CAD build for the part. Positions are in the model's coordinates, mm. Face numbers are marked on the shaded views. A direction names the side the tool comes from. Give positions to 0.01 mm unless a question says otherwise; leave off trailing zeros. Loops run counter-clockwise (first coordinate to the right, second up) from the corner with the lowest first, then second, coordinate; pieces in that order, holes last. Notation, with made-up numbers: (67, 50.5) -> (72, 50.5) arc R24 cw to (72, 61.5) -> close; hole circle Ø3 at (-4.75, 49.5). An arc over 180 degrees is marked (long way). Use one line per item in the form item = value.
```python
from build123d import *

# Parameters (mm, degrees)
CUT_EXTRUDE1_START         = -1.5875
CUT_EXTRUDE1_OUTLINE_W     = 53.975
CUT_EXTRUDE1_OUTLINE_H     = 19.05
CUT_EXTRUDE1_OUTLINE_W_2   = 50.8
CUT_EXTRUDE1_OUTLINE_H_2   = 15.875
CUT_EXTRUDE1_DEPTH         = 38.1
CUT_EXTRUDE1_START_2       = 30.1625
CUT_EXTRUDE1_2_DEPTH       = 166.6875
CUT_EXTRUDE1_3_DEPTH       = 6.35
CUT_EXTRUDE1_4_OUTLINE_W   = 50.8
CUT_EXTRUDE1_4_OUTLINE_H   = 15.875
CUT_EXTRUDE1_4_OUTLINE_W_2 = 7.9375
CUT_EXTRUDE1_4_OUTLINE_H_2 = 12.7
CUT_EXTRUDE1_4_DEPTH       = 1.5875
CUT_EXTRUDE1_5_DEPTH       = 26.9875
CUT_EXTRUDE1_6_OUTLINE_W   = 28.575
CUT_EXTRUDE1_6_OUTLINE_H   = 19.05
CUT_EXTRUDE1_6_DEPTH       = 7.9375
CUT_EXTRUDE1_START_3       = 2.38125
CUT_EXTRUDE1_7_DEPTH       = 14.2875
CUT_EXTRUDE1_8_DEPTH       = 19.05
SKETCH2_W                  = 8.89
SKETCH2_H                  = 2.5908
CUT_EXTRUDE2_DEPTH         = 203.030816028
SKETCH3_W                  = 1.9812
SKETCH3_H                  = 2.9972
CUT_EXTRUDE3_DEPTH         = 203.030816028
FILLET1_R                  = 1.5875
HOLE1_D                    = 6.35
HOLE1_DEPTH                = 1.5875


with BuildPart() as part:
    # Cut-Extrude1: read off the stored shape, not the designer's step
    # Cut-Extrude1 outline → Cut-Extrude1 (new body)
    with BuildSketch(Plane.XY.offset(-36.5125).offset(CUT_EXTRUDE1_START)):
        with Locations((14.2875, 9.525)):
            Rectangle(CUT_EXTRUDE1_OUTLINE_W, CUT_EXTRUDE1_OUTLINE_H)
        with Locations((14.2875, 9.525)):
            Rectangle(CUT_EXTRUDE1_OUTLINE_W_2, CUT_EXTRUDE1_OUTLINE_H_2, mode=Mode.SUBTRACT)
    extrude(amount=CUT_EXTRUDE1_DEPTH)

    # Cut-Extrude1 2 outline → Cut-Extrude1 2 (add)
    with BuildSketch(Plane.XY.offset(-36.5125).offset(CUT_EXTRUDE1_START_2)):
        with BuildLine():
            Line((3.175, 1.5875), (25.4, 1.5875))
            ThreePointArc((25.4, 1.5875), (26.19375, 1.800184672), (26.774815328, 2.38125))
            Line((26.774815328, 2.38125), (1.800184672, 2.38125))
            ThreePointArc((1.800184672, 2.38125), (2.38125, 1.800184672), (3.175, 1.5875))
        make_face()
    extrude(amount=CUT_EXTRUDE1_2_DEPTH)

    # Cut-Extrude1 3 outline → Cut-Extrude1 3 (add)
    with BuildSketch(Plane.XY.offset(-36.5125).offset(CUT_EXTRUDE1_START_2)):
        with BuildLine():
            Line((25.4, 1.5875), (39.6875, 1.5875))
            Line((39.6875, 1.5875), (39.6875, 17.4625))
            Line((39.6875, 17.4625), (-11.1125, 17.4625))
            Line((-11.1125, 17.4625), (-11.1125, 1.5875))
            Line((-11.1125, 1.5875), (3.175, 1.5875))
            ThreePointArc((3.175, 1.5875), (2.38125, 1.800184672), (1.800184672, 2.38125))
            Line((1.800184672, 2.38125), (3.96875, 2.38125))
            ThreePointArc((3.96875, 2.38125), (2.846217985, 2.846217985), (2.38125, 3.96875))
            Line((2.38125, 3.96875), (2.38125, 15.08125))
            ThreePointArc((2.38125, 15.08125), (2.846217985, 16.203782015), (3.96875, 16.66875))
            Line((3.96875, 16.66875), (24.60625, 16.66875))
            ThreePointArc((24.60625, 16.66875), (25.728782015, 16.203782015), (26.19375, 15.08125))
            Line((26.19375, 15.08125), (26.19375, 3.96875))
            ThreePointArc((26.19375, 3.96875), (25.728782015, 2.846217985), (24.60625, 2.38125))
            Line((24.60625, 2.38125), (26.774815328, 2.38125))
            ThreePointArc((26.774815328, 2.38125), (26.19375, 1.800184672), (25.4, 1.5875))
        make_face()
    extrude(amount=CUT_EXTRUDE1_3_DEPTH)

    # Cut-Extrude1 4 outline → Cut-Extrude1 4 (add)
    with BuildSketch(Plane.XY.offset(-36.5125).offset(CUT_EXTRUDE1_START)):
        with Locations((14.2875, 9.525)):
            Rectangle(CUT_EXTRUDE1_4_OUTLINE_W, CUT_EXTRUDE1_4_OUTLINE_H)
        with Locations((30.1625, 9.525)):
            Rectangle(CUT_EXTRUDE1_4_OUTLINE_W_2, CUT_EXTRUDE1_4_OUTLINE_H_2, mode=Mode.SUBTRACT)
    extrude(amount=CUT_EXTRUDE1_4_DEPTH)

    # Cut-Extrude1 5 outline → Cut-Extrude1 5 (add)
    with BuildSketch(Plane.XY.offset(-36.5125).offset(CUT_EXTRUDE1_START_2)):
        with BuildLine():
            Line((25.4, 17.4625), (3.175, 17.4625))
            ThreePointArc((3.175, 17.4625), (2.052467985, 16.997532015), (1.5875, 15.875))
            Line((1.5875, 15.875), (1.5875, 3.175))
            ThreePointArc((1.5875, 3.175), (1.641592751, 2.764124766), (1.800184672, 2.38125))
            Line((1.800184672, 2.38125), (3.96875, 2.38125))
            ThreePointArc((3.96875, 2.38125), (2.846217985, 2.846217985), (2.38125, 3.96875))
            Line((2.38125, 3.96875), (2.38125, 15.08125))
            ThreePointArc((2.38125, 15.08125), (2.846217985, 16.203782015), (3.96875, 16.66875))
            Line((3.96875, 16.66875), (24.60625, 16.66875))
            ThreePointArc((24.60625, 16.66875), (25.728782015, 16.203782015), (26.19375, 15.08125))
            Line((26.19375, 15.08125), (26.19375, 3.96875))
            ThreePointArc((26.19375, 3.96875), (25.728782015, 2.846217985), (24.60625, 2.38125))
            Line((24.60625, 2.38125), (26.774815328, 2.38125))
            ThreePointArc((26.774815328, 2.38125), (26.933407249, 2.764124766), (26.9875, 3.175))
            Line((26.9875, 3.175), (26.9875, 15.875))
            ThreePointArc((26.9875, 15.875), (26.522532015, 16.997532015), (25.4, 17.4625))
        make_face()
    extrude(amount=CUT_EXTRUDE1_5_DEPTH)

    # Cut-Extrude1 6 outline → Cut-Extrude1 6 (add)
    with BuildSketch(Plane.XY.offset(-36.5125).offset(CUT_EXTRUDE1_START_2)):
        with Locations((14.2875, 9.525)):
            Rectangle(CUT_EXTRUDE1_6_OUTLINE_W, CUT_EXTRUDE1_6_OUTLINE_H)
        with BuildLine():
            Line((25.4, 1.5875), (3.175, 1.5875))
            ThreePointArc((3.175, 1.5875), (2.052467985, 2.052467985), (1.5875, 3.175))
            Line((1.5875, 3.175), (1.5875, 15.875))
            ThreePointArc((1.5875, 15.875), (2.052467985, 16.997532015), (3.175, 17.4625))
            Line((3.175, 17.4625), (25.4, 17.4625))
            ThreePointArc((25.4, 17.4625), (26.522532015, 16.997532015), (26.9875, 15.875))
            Line((26.9875, 15.875), (26.9875, 3.175))
            ThreePointArc((26.9875, 3.175), (26.522532015, 2.052467985), (25.4, 1.5875))
        make_face(mode=Mode.SUBTRACT)
    extrude(amount=CUT_EXTRUDE1_6_DEPTH)

    # Cut-Extrude1 7 outline → Cut-Extrude1 7 (cut)
    with BuildSketch(Plane(origin=(0, 0, 0), x_dir=(1, 0, 0), z_dir=(0, 1, 0)).offset(CUT_EXTRUDE1_START_3)):
        Polygon((41.275, 6.35), (28.575, 0), (41.275, 0), align=None)
        Polygon((38.89375, 6.35), (-10.31875, 6.35), (6.38125, -2), (22.19375, -2), align=None)
        Polygon((0, 0), (-12.7, 6.35), (-12.7, 0), align=None)
    extrude(amount=CUT_EXTRUDE1_7_DEPTH, mode=Mode.SUBTRACT)

    # Cut-Extrude1 8 outline → Cut-Extrude1 8 (cut)
    with BuildSketch(Plane(origin=(0, 0, 0), x_dir=(1, 0, 0), z_dir=(0, 1, 0))):
        Polygon((41.275, 6.35), (28.575, 0), (41.275, 0), align=None)
        Polygon((0, 0), (-12.7, 6.35), (-12.7, 0), align=None)
    extrude(amount=CUT_EXTRUDE1_8_DEPTH, mode=Mode.SUBTRACT)

    # Sketch2 → Cut-Extrude2 (cut, through all)
    with BuildSketch(Plane.XY.offset(-36.5125)):
        with Locations((14.2875, 4.146252538)):
            Rectangle(SKETCH2_W, SKETCH2_H)
    extrude(amount=-CUT_EXTRUDE2_DEPTH, mode=Mode.SUBTRACT)

    # Sketch3 → Cut-Extrude3 (cut, through all)
    with BuildSketch(Plane.XY.offset(-36.5125)):
        with Locations((17.7419, 8.921452538)):
            Rectangle(SKETCH3_W, SKETCH3_H)
    extrude(amount=-CUT_EXTRUDE3_DEPTH, mode=Mode.SUBTRACT)

    # Fillet1
    fillet1_edges = [part.edges().sort_by_distance(p)[0] for p in [
        (-6.35, 0, -3.175),
        (-12.7, 0, -22.225),
        (-6.35, 19.05, -3.175),
        (-12.7, 9.525, -6.35),
        (-12.7, 19.05, -22.225),
        (41.275, 0, -22.225),
        (34.925, 0, -3.175),
        (41.275, 9.525, -6.35),
        (34.925, 19.05, -3.175),
        (41.275, 19.05, -22.225),
    ]]
    fillet(fillet1_edges, radius=FILLET1_R)

    # Hole1
    with Locations(Plane.XY.offset(-36.5125)):
        with Locations((-1.5875, 9.525)):
            Hole(HOLE1_D / 2, depth=HOLE1_DEPTH)


solid = part.part
```
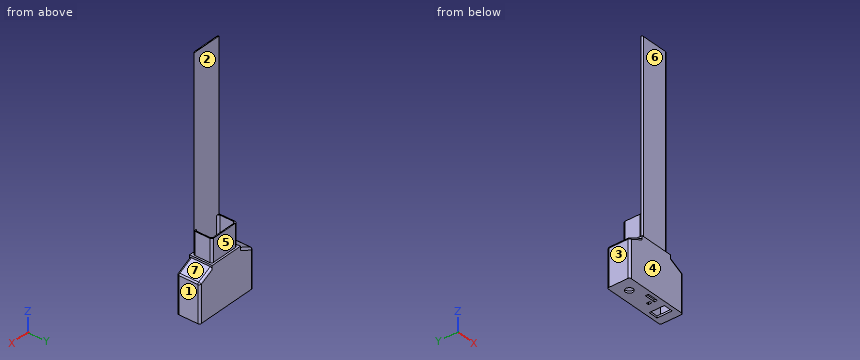
1. Drop flat-ended pins along their axis: P1, Ø10, axis at x = -1.59, y = 9.52, coming from the +Z side; P2, Ø15, axis at x = 23.5, z = 53.5, coming from the +Y side; P3, Ø5, axis at x = 22.5, y = 13, coming from the +Z side. Give the stop position or say it passes through.
Result sheet:
P1 = 20.64
P2 = 2.38
P3 = -36.51
2. Drill centre lines: line 1 (X direction, y = 2.5, z = -13) (1 decimal); line 2 (Y direction, x = 6, z = -5.5); line 3 (Z direction, x = -8, y = 6.75). Where is each one in solid material? Low to high.
Result sheet:
line_1 = -12.7 to -11.1, 39.7 to 41.3
line_2 = 0 to 2.38, 16.67 to 19.05
line_3 = -38.1 to -36.51, -5.19 to -4
3. Cut at A-A, the plane z = 89. Write the cut outline in (x, y) (1 decimal), then the cut area to 3 significant figures.
Result sheet:
outline = (1.8, 2.4) arc R1.6 ccw to (3.2, 1.6) -> (25.4, 1.6) arc R1.6 ccw to (26.8, 2.4) -> close
area = 19.2 mm^2
4. Mould opens along X. For the marked faces 1, 2, 3 and 4 say: pulls with the +X half, pulls with the -X half, needs draft (parallel to the pull), parting line crosses it, or undercut.
Result sheet:
face_1 = pulls with the +X half
face_2 = undercut
face_3 = pulls with the -X half
face_4 = needs draft
5. Tool access for the marked faces 5, 6 and 7: list every direction of +Z, -Z, +X, -X, +Y, -Y with a clear straight run to the whole face (end or side of a thin tool).
Result sheet:
face_5 = +Z, +X, -X, +Y
face_6 = +Z, +X, -X, -Y
face_7 = +Z, +X, +Y, -Y
